Geometry check sheet. Reference: the model listing, model coordinates, mm. Face numbers are marked on the shaded views. A direction names the side the tool comes from. Coordinates: 2 decimals unless noted, no trailing zeros. Order: outer loops, then holes, each group sorted by start corner. A loop starts at its lowest first (then second) coordinate and runs counter-clockwise, first axis right, second up. Notation, with made-up numbers: (-15, -0.75) - (31, -0.75) arc R25 cw to (31, 11.25) - close; hole circle Ø11 at (70, 52.5). An arc over 180 degrees is marked (long way). Return JSON: item names as keys, results as strings. Group by question number.
Item 1: Section check B-B on x = 0. Enter the section's corners in (y, z) (3 decimals), then the cut area to 3 significant figures.
Item 2: Section check C-C on z = 12. Enter the section's corners in (x, y).
Item 3: Draft check along Y on the marked faces 6, 7 and 8. Enter one of: pulls with the +Y half, pulls with the -Y half, needs draft (parallel to the pull), parting line crosses it, or undercut.
Item 4: Tool access check on the marked faces 1, 2, 3, 4 and 5. Record the directions out of +Z, -Z, +X, -X, +Y, -Y that give a thin tool (end or side, any length) a straight path to the whole face; none if there is none.
Item 5: Section check A-A on z = 0. Enter the section's corners in (x, y) (3 decimals).
Item 6: Scan lines: probe 1 along Z at (x, y) = (-16, -29.5); probe 2 along Z at (x, y) = (-12.5, -22.5); probe 3 along X at (y, z) = (-6, 0) (3 decimals). Record each from-to range of solid material in increasing order.
Item 7: Gauge pin test, flat ends, axial feed: pin 1 (1 mm diameter, centred on y = -39.5, z = 11.5, fed in from -X); pin 2 (8 mm diameter, centred on x = 7, y = -48.5, fed in from +Z); pin 3 (3 mm diameter, centred on x = 8, z = -4.5, fed in from +Y). Record the tip position at first contact, or that the pin passes through.
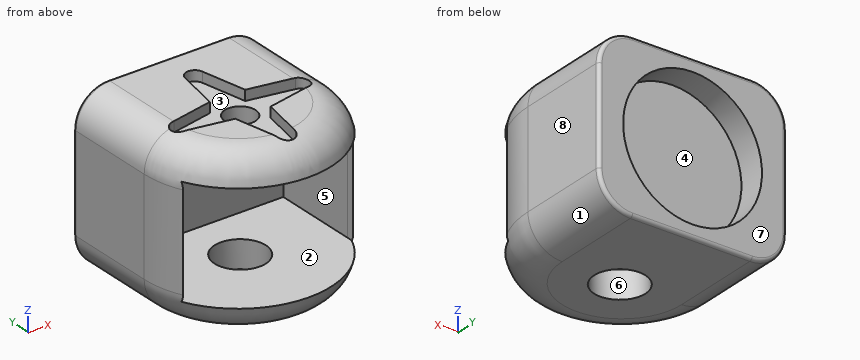
from build123d import *

# Parameters (mm, degrees)
BOSS_EXTRUDE1_DEPTH    = 24
SKETCH3_R              = 20.325
CUT_EXTRUDE1_DEPTH     = 8
FILLET1_R              = 10
FILLET5_R              = 1
CUT_EXTRUDE2_DEPTH     = 16
SKETCH10_R             = 4.5
CUT_EXTRUDE4_DEPTH     = 75
CUT_EXTRUDE5_START     = -3
CUT_EXTRUDE5_OUTLINE_R = 4.5
CUT_EXTRUDE5_DEPTH     = 3
SKETCH12_R             = 7.5
CUT_EXTRUDE6_DEPTH     = 10


# Read off the part's stored shape, not the designer's step: Cut-Extrude5
with BuildPart() as part:
    # Sketch2 → Boss-Extrude1 (new, symmetric)
    with BuildSketch(Plane.XY):
        with BuildLine():
            Line((-27.5, -27.5), (-27.5, 0))
            Line((-27.5, 0), (27.5, 0))
            Line((27.5, 0), (27.5, -27.5))
            ThreePointArc((27.5, -27.5), (0, -55), (-27.5, -27.5))
        make_face()
    extrude(amount=BOSS_EXTRUDE1_DEPTH, both=True)

    # Sketch3 → Cut-Extrude1 (cut)
    with BuildSketch(Plane(origin=(0, 0, 0), x_dir=(1, 0, 0), z_dir=(0, 1, 0))):
        with Locations(Location((0, 0, 0), (0, 0, 270))):
            Circle(SKETCH3_R)
    extrude(amount=-CUT_EXTRUDE1_DEPTH, mode=Mode.SUBTRACT)

    # Fillet1
    fillet1_edges = [part.edges().sort_by_distance(p)[0] for p in [
        (-27.5, -13.75, 24),
        (0, -55, 24),
        (-27.5, -13.75, -24),
        (27.5, -13.75, -24),
        (0, -55, -24),
        (27.5, -13.75, 24),
    ]]
    fillet(fillet1_edges, radius=FILLET1_R)

    # Fillet5
    fillet5_edges = [part.edges().sort_by_distance(p)[0] for p in [
        (27.5, 0, 0),
        (0, 0, -24),
        (-27.5, 0, 0),
        (0, 0, 24),
        (-24.571067812, 0, 21.071067812),
        (-24.571067812, 0, -21.071067812),
        (24.571067812, 0, 21.071067812),
        (24.571067812, 0, -21.071067812),
    ]]
    fillet(fillet5_edges, radius=FILLET5_R)

    # Sketch7 → Cut-Extrude2 (cut, symmetric)
    with BuildSketch(Plane.XY):
        with BuildLine():
            Line((-0.011296589, -11.876404256), (-25.011296589, -11.876404256))
            Line((-25.011296589, -11.876404256), (-25.011296589, -36.876404256))
            ThreePointArc((-25.011296589, -36.876404256), (-0.011296589, -61.876404256), (24.988703411, -36.876404256))
            Line((24.988703411, -36.876404256), (24.988703411, -11.876404256))
            Line((24.988703411, -11.876404256), (-0.011296589, -11.876404256))
        make_face()
    extrude(amount=CUT_EXTRUDE2_DEPTH, both=True, mode=Mode.SUBTRACT)

    # Sketch10 → Cut-Extrude4 (cut)
    with BuildSketch(Plane.XY.offset(24)):
        with Locations((0, -28.319318025)):
            Circle(SKETCH10_R)
    extrude(amount=-CUT_EXTRUDE4_DEPTH, mode=Mode.SUBTRACT)

    # Cut-Extrude5 outline → Cut-Extrude5 (cut)
    with BuildSketch(Plane.XY.offset(24).offset(CUT_EXTRUDE5_START)):
        with BuildLine():
            Line((-17.5, -25.637455941), (-17.5, -25.723648554))
            ThreePointArc((-17.5, -25.723648554), (-20.230845732, -28.004301665), (-18.128753541, -30.874860051))
            Line((-18.128753541, -30.874860051), (-5.197589428, -33.297375723))
            Line((-5.197589428, -33.297375723), (-2.555542026, -46.448071566))
            ThreePointArc((-2.555542026, -46.448071566), (0, -48.569318025), (2.555542026, -46.448071565))
            Line((2.555542026, -46.448071565), (4.978057698, -33.516907452))
            Line((4.978057698, -33.516907452), (18.128753541, -30.874860051))
            ThreePointArc((18.128753541, -30.874860051), (20.25, -28.319318024), (18.128753541, -25.763775998))
            Line((18.128753541, -25.763775998), (5.197589428, -23.341260326))
            Line((5.197589428, -23.341260326), (2.555542026, -10.190564483))
            ThreePointArc((2.555542026, -10.190564483), (0, -8.069318025), (-2.555542026, -10.190564483))
            Line((-2.555542026, -10.190564483), (-4.978057698, -23.121728597))
            Line((-4.978057698, -23.121728597), (-17.5, -25.637455941))
        make_face()
        with Locations((0, -28.319318025)):
            Circle(CUT_EXTRUDE5_OUTLINE_R, mode=Mode.SUBTRACT)
    extrude(amount=CUT_EXTRUDE5_DEPTH, mode=Mode.SUBTRACT)

    # Sketch12 → Cut-Extrude6 (cut)
    with BuildSketch(Plane(origin=(0, 0, -24), x_dir=(-1, 0, 0), z_dir=(0, 0, -1))):
        with Locations((0, -28.319318025)):
            Circle(SKETCH12_R)
    extrude(amount=-CUT_EXTRUDE6_DEPTH, mode=Mode.SUBTRACT)


solid = part.part
Computed:
{
 "1": {"outline": "(-54.798, -16) arc R10 ccw to (-45, -24) - (-35.819, -24) - (-35.819, -16) - close; (-54.798, 16) - (-32.819, 16) - (-32.819, 21) - (-48.569, 21) - (-48.569, 23.341) arc R10 ccw to start; (-23.819, 16) - (-11.876, 16) - (-11.876, -16) - (-20.819, -16) - (-20.819, -24) - (-1, -24) arc R1 ccw to (0, -23) - (0, -20.325) - (-8, -20.325) - (-8, 20.325) - (0, 20.325) - (0, 23) arc R1 ccw to (-1, 24) - (-8.069, 24) - (-8.069, 21) - (-23.819, 21) - close", "area": "606 mm²"},
 "2": {"outline": "(-27.5, -27.5) arc R27.5 ccw to (-24.91, -39.16) arc R25 cw to (-25.01, -36.88) - (-25.01, -11.88) - (24.99, -11.88) - (24.99, -36.88) arc R25 cw to (24.88, -39.22) arc R27.5 ccw to (27.5, -27.5) - (27.5, -1) arc R1 ccw to (26.5, 0) - (16.4, 0) - (16.4, -8) - (-16.4, -8) - (-16.4, 0) - (-26.5, 0) arc R1 ccw to (-27.5, -1) - close"},
 "3": {"face 6": "undercut", "face 7": "pulls with the +Y half", "face 8": "needs draft"},
 "4": {"face 1": "-Z, +X, +Y, -Y", "face 2": "-Y", "face 3": "+Z", "face 4": "+Y", "face 5": "none"},
 "5": {"outline": "(-27.5, -27.5) arc R27.5 ccw to (-24.907, -39.157) arc R25 cw to (-25.011, -36.876) - (-25.011, -11.876) - (24.989, -11.876) - (24.989, -36.876) arc R25 cw to (24.879, -39.217) arc R27.5 ccw to (27.5, -27.5) - (27.5, -1) arc R1 ccw to (26.5, 0) - (20.325, 0) - (20.325, -8) - (-20.325, -8) - (-20.325, 0) - (-26.5, 0) arc R1 ccw to (-27.5, -1) - close"},
 "6": {"probe 1": "z = -24 to -16, 16 to 21", "probe 2": "z = -24 to -16, 16 to 24", "probe 3": "x = -27.5 to -20.325, 20.325 to 27.5"},
 "7": {"pin 1": "stops at x = -24.98", "pin 2": "stops at z = 23.98", "pin 3": "stops at y = -8"}
}
